Could you check a few things on this model? Use its own coordinates, in mm. A direction names the side the tool comes from. Coordinates: 2 decimals unless noted, no trailing zeros. Write each loop counter-clockwise with the first axis right and the second up, starting at its lowest first coordinate (ties: lowest second). Pieces come first, ordered by that corner, then holes. Notation, with made-up numbers: (60.5, 7.25) - (82.5, 7.25) arc R10 cw to (82.5, 26.25) - close; hole circle Ø10 at (1, 53.5). An arc over 180 degrees is marked (long way). Answer as a JSON object with one key per item and string values. Group by question number.
1) Please list where these lines run through material, in increasing order: line 1 along X through (y, z) = (-14.7, -5); line 2 along X through (y, z) = (-2, -18); line 3 along Y through (x, z) = (4.5, -0.65).
2) If we section it at D-D (x = -12): Write out the boundary of the cut face in (y, z), plus the area to 3 significant figures.
3) We'd pull the mould along Z, two halves only. Please class faces 1 (the flat face through (0, -20, -20)), 2 (the cylindrical face through (12.466, -14.754, -38.478)), 3 (the flat face through (-2, -16, -40)): released by +Z, released by -Z, zero draft, split by the parting line, or undercut.
4) If we section it at C-C (y = -15.5): Write out the boundary of the cut face in (x, z).
5) On a 3-axis mill with a long thin cutter (end or side, diameter ignored), from which of +Z, -Z, +X, -X, +Y, -Y can I reach the whole of each face in a straight line? I mean faces 4 (the flat face through (14.5, 0, -21)), 5 (the cylindrical face through (3.59, 8.6, -0.99)), 6 (the cylindrical face through (-11.534, -14.754, -38.478)). Say none if no direction works.
6) Will these pins go through, and if not, where does the flat tip stop? pin 1 Ø3 at (x, z) = (-4.5, -16.5) entering from +Y; pin 2 Ø5.5 at (x, y) = (-4.5, -10.04) entering from -Z.
7) If we section it at B-B (x = 0): Write out the boundary of the cut face in (y, z), plus the area to 3 significant figures.
8) If we section it at A-A (z = -5): State how many separate pieces and enclosed holes the cut face has, plus the area to 3 significant figures.
```python
from build123d import *

# Parameters (mm, degrees)
SKETCH1_W                                            = 30
SKETCH1_H                                            = 30
BOSS_EXTRUDE1_DEPTH                                  = 40
SKETCH7_W                                            = 29
SKETCH7_H                                            = 29
CUT_EXTRUDE5_DEPTH                                   = 38
CSK_FOR_M3_CROSS_COUNTERSUNK_HEAD_SCREW1_D           = 3.4
CSK_FOR_M3_CROSS_COUNTERSUNK_HEAD_SCREW1_CSINK_D     = 6
CSK_FOR_M3_CROSS_COUNTERSUNK_HEAD_SCREW1_CSINK_ANGLE = 92
SKETCH18_W                                           = 30
SKETCH18_H                                           = 40
CUT_EXTRUDE6_DEPTH                                   = 1
SKETCH19_R                                           = 1.55
CUT_EXTRUDE7_DEPTH                                   = 1
CUT_EXTRUDE8_DEPTH                                   = 46.276925691
CUT_EXTRUDE8_DEPTH_BACK                              = 46.276925691
SKETCH20_R                                           = 8.2177971
SKETCH22_R                                           = 1.5
SKETCH22_R_2                                         = 1.517998986
BOSS_EXTRUDE2_DEPTH                                  = 5


with BuildPart() as part:
    # Sketch1 → Boss-Extrude1 (new body)
    with BuildSketch(Plane.XY):
        Rectangle(SKETCH1_W, SKETCH1_H)
    extrude(amount=-BOSS_EXTRUDE1_DEPTH)

    # Sketch7 → Cut-Extrude5 (cut)
    with BuildSketch(Plane(origin=(0, 0, -40), x_dir=(-1, 0, 0), z_dir=(0, 0, -1))):
        Rectangle(SKETCH7_W, SKETCH7_H)
    extrude(amount=-CUT_EXTRUDE5_DEPTH, mode=Mode.SUBTRACT)

    # CSK for M3 Cross Countersunk Head Screw1 (through all)
    with Locations(Plane(origin=(0, 0, -40), x_dir=(1, 0, 0), z_dir=(0, 0, -1))):
        with Locations((-4.5, -10.03742995), (4.5, -10.03742995), (4.5, 10.03742995), (-4.5, 10.03742995)):
            CounterSinkHole(CSK_FOR_M3_CROSS_COUNTERSUNK_HEAD_SCREW1_D / 2, CSK_FOR_M3_CROSS_COUNTERSUNK_HEAD_SCREW1_CSINK_D / 2, counter_sink_angle=CSK_FOR_M3_CROSS_COUNTERSUNK_HEAD_SCREW1_CSINK_ANGLE)

    # Sketch18 → Cut-Extrude6 (cut)
    with BuildSketch(Plane(origin=(0, 15, 0), x_dir=(1, 0, 0), z_dir=(0, 1, 0))):
        with Locations((0, 20)):
            Rectangle(SKETCH18_W, SKETCH18_H)
    extrude(amount=-CUT_EXTRUDE6_DEPTH, mode=Mode.SUBTRACT)

    # Sketch19 → Cut-Extrude7 (cut)
    with BuildSketch(Plane.XZ.offset(15)):
        with Locations(Location((-12, -5, 0), (0, 0, 270))):
            Circle(SKETCH19_R)
        with Locations(Location((-12, -37, 0), (0, 0, 270))):
            Circle(SKETCH19_R)
        with Locations(Location((12, -37, 0), (0, 0, 270))):
            Circle(SKETCH19_R)
        with Locations(Location((12, -5, 0), (0, 0, 270))):
            Circle(SKETCH19_R)
    extrude(amount=-CUT_EXTRUDE7_DEPTH, mode=Mode.SUBTRACT)

    # Sketch20 → Cut-Extrude8 (cut, two sides: drawn at the far end of the back side and taken through both)
    with BuildSketch(Plane.XY.offset(-CUT_EXTRUDE8_DEPTH_BACK)):
        Circle(SKETCH20_R)
    extrude(amount=CUT_EXTRUDE8_DEPTH + CUT_EXTRUDE8_DEPTH_BACK, mode=Mode.SUBTRACT)

    # Sketch22 → Boss-Extrude2 (add)
    with BuildSketch(Plane.XZ.offset(15)):
        Polygon((15, -40), (14.5, -40), (-14.5, -40), (-15, -40), (-15, 0), (15, 0), align=None)
        with Locations(Location((-12, -5, 0), (0, 0, 270))):
            Circle(SKETCH22_R, mode=Mode.SUBTRACT)
        with Locations(Location((12, -5, 0), (0, 0, 270))):
            Circle(SKETCH22_R_2, mode=Mode.SUBTRACT)
        with Locations(Location((-12, -37, 0), (0, 0, 270))):
            Circle(SKETCH22_R, mode=Mode.SUBTRACT)
        with Locations(Location((12, -37, 0), (0, 0, 270))):
            Circle(SKETCH22_R, mode=Mode.SUBTRACT)
    extrude(amount=BOSS_EXTRUDE2_DEPTH)


solid = part.part
```
Here are the results:
{
 "1": {"line 1": "x = -15 to -13.55, -10.45 to 10.45, 13.55 to 15", "line 2": "x = -15 to -14.5, 14.5 to 15", "line 3": "y = -20 to -11.74, -8.34 to -6.88, 6.88 to 8.34, 11.74 to 14"},
 "2": {"outline": "(-20, -40) - (-14.5, -40) - (-14.5, -38.55) - (-15, -38.55) - (-15, -38.5) - (-20, -38.5) - close; (-20, -35.5) - (-15, -35.5) - (-15, -35.45) - (-14.5, -35.45) - (-14.5, -6.55) - (-15, -6.55) - (-15, -6.5) - (-20, -6.5) - close; (-20, -3.5) - (-15, -3.5) - (-15, -3.45) - (-14.5, -3.45) - (-14.5, -2) - (14, -2) - (14, 0) - (-20, 0) - close", "area": "244 mm²"},
 "3": {"face 1": "zero draft", "face 2": "undercut", "face 3": "released by -Z"},
 "4": {"outline": "(-15, -40) - (15, -40) - (15, 0) - (-15, 0) - close; hole circle Ø3 at (-12, -37); hole circle Ø3 at (-12, -5); hole circle Ø3.04 at (12, -5); hole circle Ø3 at (12, -37)"},
 "5": {"face 4": "-Z, +Y", "face 5": "+Z, -Z", "face 6": "+Y"},
 "6": {"pin 1": "stops at y = -14.5", "pin 2": "stops at z = -2"},
 "7": {"outline": "(-20, -40) - (-14.5, -40) - (-14.5, -2) - (-8.22, -2) - (-8.22, 0) - (-20, 0) - close; (8.22, -2) - (14, -2) - (14, 0) - (8.22, 0) - close", "area": "244 mm²"},
 "8": {"separate pieces": "3", "enclosed holes": "0", "area": "160 mm²"}
}
